Here's how the part is built. I have some questions about the finished solid (model axes, mm). A direction names the side the tool comes from. Round coordinates to 2 decimals unless told otherwise and drop trailing zeros. Write each loop counter-clockwise with the first axis right and the second up, starting at its lowest first coordinate (ties: lowest second). Pieces come first, ordered by that corner, then holes. Notation, with made-up numbers: (66, -31) -> (86, -31) arc R17 cw to (86, -11) -> close; hole circle Ø3 at (58.5, 87). An arc over 180 degrees is marked (long way). Answer in a Markdown table with one row per item.
from build123d import *

# Parameters (mm, degrees)
SKETCH1_R           = 3.5
BOSS_EXTRUDE1_DEPTH = 12.7
CUT_EXTRUDE1_DEPTH  = 6.93
SKETCH3_R           = 1.5
CUT_EXTRUDE2_DEPTH  = 6.77
SKETCH4_R           = 2
CUT_EXTRUDE3_DEPTH  = 10
SKETCH5_W           = 2
SKETCH5_H           = 0.5
BOSS_EXTRUDE2_DEPTH = 12.7
FILLET1_R           = 3.175
SKETCH6_R           = 1.585
CUT_EXTRUDE4_DEPTH  = 1.5


with BuildPart() as part:
    # Sketch1 → Boss-Extrude1 (new body)
    with BuildSketch(Plane(origin=(0, 0, 0), x_dir=(1, 0, 0), z_dir=(0, 1, 0))):
        Circle(SKETCH1_R)
        with BuildLine():
            ThreePointArc((1.802775638, 3), (3.046285831, 1.723410176), (3.5, 0))
            Line((3.5, 0), (23.330212793, 0))
            Line((23.330212793, 0), (23.330212793, 3))
            Line((23.330212793, 3), (1.802775638, 3))
        make_face()
    extrude(amount=BOSS_EXTRUDE1_DEPTH)

    # Sketch2 → Cut-Extrude1 (cut)
    with BuildSketch(Plane(origin=(0, 12.7, 0), x_dir=(1, 0, 0), z_dir=(0, 1, 0))):
        with BuildLine():
            ThreePointArc((6.330212793, 3), (-6.149926342, 1.5), (6.330212793, 0))
            Line((6.330212793, 0), (3.5, 0))
            ThreePointArc((3.5, 0), (-3.046285831, -1.723410176), (1.802775638, 3))
            Line((1.802775638, 3), (6.330212793, 3))
        make_face()
        with BuildLine():
            Line((3.5, 0), (6.330212793, 0))
            ThreePointArc((6.330212793, 0), (4.830212793, 1.5), (6.330212793, 3))
            Line((6.330212793, 3), (1.802775638, 3))
            ThreePointArc((1.802775638, 3), (-3.046285831, -1.723410176), (3.5, 0))
        make_face()
    extrude(amount=-CUT_EXTRUDE1_DEPTH, mode=Mode.SUBTRACT)

    # Sketch3 → Cut-Extrude2 (cut, through all)
    with BuildSketch(Plane(origin=(0, 5.77, 0), x_dir=(1, 0, 0), z_dir=(0, 1, 0))):
        with Locations(Location((0, 0, 0), (0, 0, 270))):  # turned: the seam where the file's is
            Circle(SKETCH3_R)
    extrude(amount=-CUT_EXTRUDE2_DEPTH, mode=Mode.SUBTRACT)


with BuildPart() as body_2:
    # Mirror1: mirrored copy
    add(part.part.mirror(Plane.XY.offset(-5)))

    # Sketch4 → Cut-Extrude3 (cut)
    with BuildSketch(Plane.XY.offset(-7)):
        with Locations((59.285262001, -42.831378851)):
            Circle(SKETCH4_R)
        with Locations((59.285262001, -47.531378851)):
            Circle(SKETCH4_R)
    extrude(amount=-CUT_EXTRUDE3_DEPTH, mode=Mode.SUBTRACT)

    # Sketch5 → Boss-Extrude2 (add)
    with BuildSketch(Plane(origin=(0, 12.7, 0), x_dir=(1, 0, 0), z_dir=(0, 1, 0))):
        with BuildLine():
            Line((21.330212793, 6.5), (21.330212793, 7))
            Line((21.330212793, 7), (19.59096008, 7))
            ThreePointArc((19.59096008, 7), (20.495808134, 6.872518864), (21.330212793, 6.5))
        make_face()
        with Locations((22.330212793, 6.75)):
            Rectangle(SKETCH5_W, SKETCH5_H)
    extrude(amount=-BOSS_EXTRUDE2_DEPTH)

    # Fillet1
    fillet1_edges = [body_2.edges().sort_by_distance(p)[0] for p in [
        (1.802775638, 2.885, -7),
        (3.5, 2.885, -10),
        (23.330212793, 6.35, -10),
    ]]
    fillet(fillet1_edges, radius=FILLET1_R)

    # Sketch6 → Cut-Extrude4 (cut)
    with BuildSketch(Plane.XY.offset(-7)):
        with Locations((66.743933259, -45.181378851)):
            Circle(SKETCH6_R)
    extrude(amount=-CUT_EXTRUDE4_DEPTH, mode=Mode.SUBTRACT)


solid = body_2.part
1) For pin 1 (1 mm diameter, centred on y = 3, z = -11, fed in from +X); pin 2 (4 mm diameter, centred on x = 11.5, y = 4.5, fed in from -Z); pin 3 (4 mm diameter, centred on x = 13.5, y = 3, fed in from +Z), each with a flat end and sliding along its axis, tell me the tip position at first contact or that it passes through.
Response:
| item | result |
|---|---|
| pin 1 | stops at x = 4.16 |
| pin 2 | stops at z = -10 |
| pin 3 | stops at z = -7 |
2) I want a section at D-D, the plane y = 8. List the corners of the cut face in (x, z) for me (3 decimals).
Response:
| item | result |
|---|---|
| outline | (6.33, -10) -> (20.155, -10) arc R3.175 ccw to (23.33, -6.825) -> (23.33, -6.5) -> (21.33, -6.5) arc R3.275 cw to (19.591, -7) -> (6.33, -7) arc R1.5 ccw to start |
3) I want a section at A-A, the plane x = 0. List the corners of the cut face in (y, z) for me, and give its area (3 significant figures).
Response:
| item | result |
|---|---|
| outline | (0, -13.5) -> (5.77, -13.5) -> (5.77, -11.5) -> (0, -11.5) -> close; (0, -8.5) -> (5.77, -8.5) -> (5.77, -6.5) -> (0, -6.5) -> close |
| area | 23.1 mm^2 |
4) I want a section at C-C, the plane z = -11.25. List the corners of the cut face in (x, y) for me.
Response:
| item | result |
|---|---|
| outline | (-3.27, 0) -> (-0.83, 0) -> (-0.83, 5.77) -> (-3.27, 5.77) -> close; (0.83, 0) -> (3.35, 0) -> (3.35, 5.77) -> (0.83, 5.77) -> close |
5) I want a section at B-B, the plane y = 4.5. List the corners of the cut face in (x, z) for me (3 decimals), and give its area (3 significant figures).
Response:
| item | result |
|---|---|
| outline | (1.329, -6.762) arc R3.5 ccw (long way) to (3.079, -11.665) arc R3.175 cw to (5.872, -10) -> (20.155, -10) arc R3.175 ccw to (23.33, -6.825) -> (23.33, -6.5) -> (21.33, -6.5) arc R3.275 cw to (19.591, -7) -> (2.535, -7) arc R3.175 cw to start; hole circle Ø3 at (0, -10) |
| area | 92.4 mm^2 |
6) I need wall thicknesses on line 1 (Y direction, x = 2.5, z = -7.5); line 2 (Z direction, x = 17.25, y = 3); line 3 (Z direction, x = 1, y = 2). Which ranges of each line are inside material? Lowest first, please. Write a range as [from, to].
Response:
| item | result |
|---|---|
| line 1 | y = [0, 5.77] |
| line 2 | z = [-10, -7] |
| line 3 | z = [-13.35, -11.12], [-8.88, -6.65] |
7) Which directions (+Z, -Z, +X, -X, +Y, -Y) give clear straight access to the entire face, cutting with the end or side of a thin tool? Please do faces 1 (the face through (1.912, 2.925, -6.938)), 2 (the face through (14, 12.7, -8)), 3 (the face through (4.83, 9.28, -8.53)).
Response:
| item | result |
|---|---|
| face 1 | +Z, +Y, -Y |
| face 2 | +Z, -Z, +X, -X, +Y |
| face 3 | -X, +Y |
8) We'd pull the mould along X, two halves only. Please class faces 4 (the face through (22.38, 6.44, -9.09)), 5 (the face through (20.483, 6.439, -6.876)), 6 (the face through (11, 6, -7)), 7 (the face through (13, 6, -10)): +X half, -X half, draft (parallel to the pull), parting line (faces both ways), or undercut.
Response:
| item | result |
|---|---|
| face 4 | +X half |
| face 5 | undercut |
| face 6 | undercut |
| face 7 | draft |
